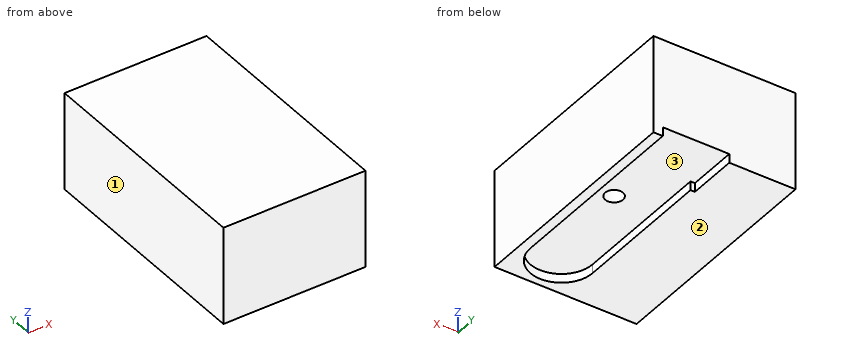
from build123d import *

# Parameters (mm, degrees)
F1_DEPTH = 11
F2_R     = 1
F3_DEPTH = 1
F4_DEPTH = 3.9


with BuildPart() as f1:
    # F0 (on Top) → F1 (new body)
    with BuildSketch(Plane.XY):
        Polygon((-7.970938, -12.932724), (8.029062, -12.932724), (8.029062, 13.067276), (4.129676, 13.067276), (0.029062, 13.067276), (-7.970938, 13.067276), align=None)
    extrude(amount=F1_DEPTH)

    # F2 (on Top) → F3 (cut)
    with BuildSketch(Plane.XY):
        with BuildLine():
            Line((-0.023847, 7.43662), (-0.023847, -8.600051))
            ThreePointArc((-0.023847, -8.600051), (3.476153, -12.100051), (6.976153, -8.600051))
            Line((6.976153, -8.600051), (6.976153, 15.099979))
            Line((6.976153, 15.099979), (-0.516003, 14.27335))
            Line((-0.516003, 14.27335), (-0.516003, 7.43662))
            Line((-0.516003, 7.43662), (-0.023847, 7.43662))
        make_face()
        with Locations((4.481404, 1.478317)):
            Circle(F2_R, mode=Mode.SUBTRACT)
        with Locations((4.481404, 1.478317)):
            Circle(F2_R)
    extrude(amount=F3_DEPTH, mode=Mode.SUBTRACT)

    # F2 (on Top) → F4 (cut)
    with BuildSketch(Plane.XY):
        with Locations((4.481404, 1.478317)):
            Circle(F2_R)
    extrude(amount=F4_DEPTH, mode=Mode.SUBTRACT)


solid = f1.part
The listing builds one solid part. Answer for the finished solid, in the listing's coordinates (mm). Face numbers are marked on the shaded views. Give positions to 0.01 mm unless a question says otherwise; leave off trailing zeros. Write each loop counter-clockwise with the first axis right and the second up, starting at its lowest first coordinate (ties: lowest second). Pieces come first, ordered by that corner, then holes.
1) Section D-D (x = 6.25) is taken. Write down the section's boundary in (y, z).
2) Find the intervals of material crossed by L1, parallel to X at y = -1.75, z = 0.75; L2, parallel to Z at x = 1.75, y = -2.75; L3, parallel to Z at x = 4, y = 1.5, in increasing order.
3) Section B-B (x = 4.5) is taken. Write down the section's boundary in (y, z).
4) Given P1, Ø1.8, axis at x = 4.48, y = 1.48, coming from the -Z side; P2, Ø3, axis at x = -5.5, y = 8.5, coming from the -Z side; P3, Ø0.6, axis at x = 5, y = 2, coming from the -Z side, each flat-ended and moving along its own axis, determine where each tip first touches the part or whether it passes through.
5) For a pull along X with two mould halves and no side action, classify the marked faces 1, 2 and 3 as pulls with the +X half, pulls with the -X half, needs draft (parallel to the pull), parting line crosses it, or undercut.
6) Section A-A (y = -6.5) is taken. Write down the section's boundary in (x, z), and give its area (3 significant figures).
7) Section C-C (y = -11) is taken. Write down the section's boundary in (x, z), and give its area (3 significant figures).
Response:
1. outline: (-12.93, 0) - (-10.73, 0) - (-10.73, 1) - (13.07, 1) - (13.07, 11) - (-12.93, 11) - close
2. L1: x = -7.97 to -0.02, 6.98 to 8.03
2. L2: z = 1 to 11
2. L3: z = 3.9 to 11
3. outline: (-12.93, 0) - (-11.95, 0) - (-11.95, 1) - (0.48, 1) - (0.48, 3.9) - (2.48, 3.9) - (2.48, 1) - (13.07, 1) - (13.07, 11) - (-12.93, 11) - close
4. P1: stops at z = 3.9
4. P2: stops at z = 0
4. P3: stops at z = 1
5. face 1: pulls with the -X half
5. face 2: needs draft
5. face 3: undercut
6. outline: (-7.97, 0) - (-0.02, 0) - (-0.02, 1) - (6.98, 1) - (6.98, 0) - (8.03, 0) - (8.03, 11) - (-7.97, 11) - close
6. area: 169 mm2
7. outline: (-7.97, 0) - (0.93, 0) - (0.93, 1) - (6.02, 1) - (6.02, 0) - (8.03, 0) - (8.03, 11) - (-7.97, 11) - close
7. area: 171 mm2
